```python
from build123d import *

# Parameters (mm, degrees)
F0_W     = 5.842
F0_H     = 12.7
F0_R     = 3.175
F3_DEPTH = 6.35


with BuildPart() as f1:
    # F0 (on Front) → F1 (revolve)
    with BuildSketch(Plane.XZ):
        with Locations((2.921, 6.35)):
            Rectangle(F0_W, F0_H)
    revolve(axis=Axis((33.147, 0, 0), (-1, 0, 0)))

    # F0 (on Front) → F2 (revolve)
    with BuildSketch(Plane.XZ):
        Polygon((5.842, 12.7), (5.842, 0), (66.294, 0), (66.294, 12.7), (56.134, 12.7), (56.134, 10.16), (10.16, 10.16), (10.16, 12.7), align=None)
    revolve(axis=Axis((33.147, 0, 0), (-1, 0, 0)))

    # F0 (on Front) → F3 (join)
    with BuildSketch(Plane.XZ):
        with BuildLine():
            ThreePointArc((-8.182663, -5.506983), (-3.195791, -4.549339), (-0.9398, 0))
            ThreePointArc((-0.9398, 0), (-4.591961, 5.329721), (-10.88063, 3.847543))
            ThreePointArc((-10.88063, 3.847543), (-12.145978, -1.583727), (-8.182663, -5.506983))
        make_face()
        with Locations((-6.6548, 0)):
            Circle(F0_R, mode=Mode.SUBTRACT)
        with BuildLine():
            Line((5.842, 0), (0, 0))
            Line((0, 0), (-0.9398, 0))
            ThreePointArc((-0.9398, 0), (-3.195791, -4.549339), (-8.182663, -5.506983))
            Line((-8.182663, -5.506983), (5.842, -9.398))
            Line((5.842, -9.398), (5.842, 0))
        make_face()
    extrude(amount=F3_DEPTH)


solid = f1.part
```
For this review, take the finished solid that the model builds, in its own axes (mm). A direction names the side the tool comes from. Give positions to 0.01 mm unless a question says otherwise; leave off trailing zeros. Write each loop counter-clockwise with the first axis right and the second up, starting at its lowest first coordinate (ties: lowest second). Pieces come first, ordered by that corner, then holes.
Item 1: Insertion check: P1, Ø6, axis at x = 48.5, y = -6.5, coming from the +Z side; P2, Ø6, axis at x = -4, z = -2, coming from the -Y side; P3, Ø10, axis at x = 1.5, z = 5.5, coming from the -Y side. Each pin has a flat end and moves straight along its axis. Give the tip position at first contact, or say it passes through.
Item 2: Take a section at C-C (z = 8). Give the boundary of the cut face in (x, y), and give its area (3 significant figures).
Item 3: Take a section at D-D (y = -1.5). Give the boundary of the cut face in (x, z) (3 decimals).
Item 4: Take a section at A-A (y = 11.25). Give the boundary of the cut face in (x, z), and give its area (3 significant figures).
Item 5: Wall thickness on probe 1 along X at (y, z) = (11.25, 3.5); probe 2 along X at (y, z) = (-3.25, 2.5); probe 3 along X at (y, z) = (-8, 2): over which ranges is each line inside the solid? List them lowest first.
Item 6: Take a section at B-B (z = -11). Give the boundary of the cut face in (x, y).
Item 7: The part is to be moulded in two halves that separate along Z. For faces 1 (the face through (-4.149, -3.131, -6.626)), 2 (the face through (5.01, -12.4, -2.75)), 3 (the face through (10.16, 9, 6)), 4 (the face through (-3.626, -3.131, 0.954)), say which applies: +Z half, -Z half, draft (parallel to the pull), parting line (faces both ways), or undercut.
Item 8: Machinability: for faces 5 (the face through (66.294, 0, 0)), 6 (the face through (-3.5, -6.35, -2.4)), 7 (the face through (61.14, -12.4, -2.75)), 8 (the face through (-3.5, 0, -2.4)), 9 (the face through (32.825, 10.074, -1.323)), which of the approach directions +Z, -Z, +X, -X, +Y, -Y give a long, thin tool a straight path to every point of the face, cutting with its end or side? Answer none if there is none.
Established:
1. P1: stops at z = 9.54
1. P2: stops at y = -6.35
1. P3: stops at y = -12.69
2. outline: (0, -9.86) - (10.16, -9.86) - (10.16, -6.26) - (56.13, -6.26) - (56.13, -9.86) - (66.29, -9.86) - (66.29, 9.86) - (56.13, 9.86) - (56.13, 6.26) - (10.16, 6.26) - (10.16, 9.86) - (0, 9.86) - close
2. area: 977 mm2
3. outline: (-8.183, -5.507) - (0, -7.777) - (0, -12.611) - (10.16, -12.611) - (10.16, -10.049) - (56.134, -10.049) - (56.134, -12.611) - (66.294, -12.611) - (66.294, 12.611) - (56.134, 12.611) - (56.134, 10.049) - (10.16, 10.049) - (10.16, 12.611) - (0, 12.611) - (0, 0) - (-0.94, 0) arc R5.715 ccw (long way) to start; hole circle Ø6.35 at (-6.655, 0)
4. outline: (0, -5.89) - (10.16, -5.89) - (10.16, 5.89) - (0, 5.89) - close; (56.13, -5.89) - (66.29, -5.89) - (66.29, 5.89) - (56.13, 5.89) - close
4. area: 239 mm2
5. probe 1: x = 0 to 10.16, 56.13 to 66.29
5. probe 2: x = -11.79 to -8.61, -4.7 to -1.52, 0 to 66.29
5. probe 3: x = 0 to 66.29
6. outline: (0, -6.35) - (10.16, -6.35) - (10.16, 6.35) - (0, 6.35) - close; (56.13, -6.35) - (66.29, -6.35) - (66.29, 6.35) - (56.13, 6.35) - close
7. face 1: -Z half
7. face 2: parting line
7. face 3: draft
7. face 4: undercut
8. face 5: +Z, -Z, +X, +Y, -Y
8. face 6: +Z, -Z, -X, -Y
8. face 7: +X, -X
8. face 8: +Z, -Z, -X, +Y
8. face 9: none
